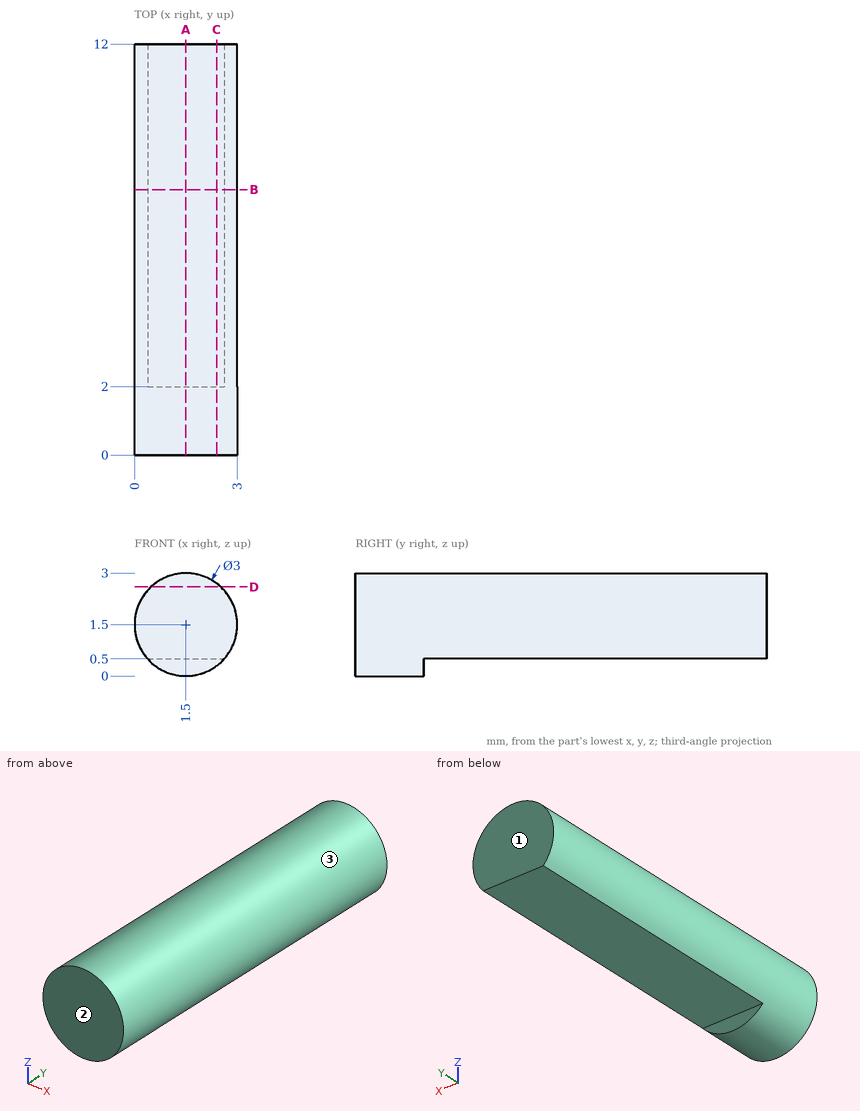
Here's the drawing with two shaded views (mm, measured from the low corner). I have some questions. Coordinates: 2 decimals unless noted, no trailing zeros. Order: outer loops, then holes, each group sorted by start corner. A loop starts at its lowest first (then second) coordinate and runs counter-clockwise, first axis right, second up. Notation, with made-up numbers: (87.25, 10.25) - (118.25, 10.25) arc R22 cw to (118.25, 17.25) - close; hole circle Ø2 at (17, 61.5). An arc over 180 degrees is marked (long way). Use CSV: the item, a comma, the result in double quotes. Start each with the question number.
1. Suppose I cut it at D-D on z = 2.6. List the corners of the cut face in (x, y) for me, then the cut area to 3 significant figures.
2. I'm going to push a flat-ended pin straight in: pin 1 (1.1 mm diameter, centred on x = 1, y = 9, fed in from -Z). Where does the tip first touch, or does it pass through?
3. Suppose I cut it at A-A on x = 1.5. List the corners of the cut face in (y, z) for me.
4. Suppose I cut it at C-C on x = 2.4. List the corners of the cut face in (y, z) for me, then the cut area to 3 significant figures.
5. Please list where these lines run through material, in increasing order: line 1 (Y direction, x = 1.3, z = 0.3); line 2 (Z direction, x = 1.55, y = 3.5); line 3 (X direction, y = 8.25, z = 2.6). Write a range as from..to.
6. If we mould it in two halves opening along Y, with no side actions, what happens to the marked faces 1, 2 and 3? For each: +Y half, -Y half, draft (parallel to the pull), parting line (faces both ways), or undercut.
7. Suppose I cut it at B-B on y = 7.75. List the corners of the cut face in (x, z) for me, then the cut area to 3 significant figures.
Output:
1,outline,"(0.48, 0) - (2.52, 0) - (2.52, 12) - (0.48, 12) - close"
1,area,"24.5 mm2"
2,pin 1,"stops at z = 0.5"
3,outline,"(0, 0) - (2, 0) - (2, 0.5) - (12, 0.5) - (12, 3) - (0, 3) - close"
4,outline,"(0, 0.3) - (2, 0.3) - (2, 0.5) - (12, 0.5) - (12, 2.7) - (0, 2.7) - close"
4,area,"26.8 mm2"
5,line 1,"y = 0..2"
5,line 2,"z = 0.5..3"
5,line 3,"x = 0.48..2.52"
6,face 1,"+Y half"
6,face 2,"-Y half"
6,face 3,"draft"
7,outline,"(0.38, 0.5) - (2.62, 0.5) arc R1.5 ccw (long way) to start"
7,area,"6.29 mm2"
